Autodesk Inventor part; units mm, degrees
ref_plane "YZ Plane" through (0, 0, 0) normal (1, 0, 0) x (0, 1, 0)
ref_plane "XZ Plane" through (0, 0, 0) normal (0, 1, 0) x (-1, 0, 0)
ref_plane "XY Plane" through (0, 0, 0) normal (0, 0, 1) x (1, 0, 0)
sketch "Sketch1" plane through (0, 0, 0) normal (0, 0, 1) x (1, 0, 0)
  line L0 (0, 0) -> (-76.2, 0)
  line L1 (-76.2, 0) -> (-76.2, 3.175)
  line L2 (-76.2, 3.175) -> (-3.175, 3.175)
  line L3 (-3.175, 3.175) -> (-3.175, 53.975)
  line L4 (-3.175, 53.975) -> (0, 53.975)
  line L5 (0, 53.975) -> (0, 0)
  dimension "d0" = 76.2
  dimension "d1" = 50.8
  dimension "d2" = 3.175
extrude "Extrusion1" add sketch "Sketch1" along normal blind 60
sketch "Sketch2" plane through (-76.2, 3.175, 0) normal (0, 1, 0) x (1, 0, 0)
  line L0 (10.98, -50) -> (63.98, -50) construction
  line L1 (63.98, -50) -> (63.98, -10) construction
  line L2 (63.98, -10) -> (10.98, -10) construction
  line L3 (10.98, -10) -> (10.98, -50) construction
  line L4 (0, 0) -> (0, -60) construction
  line L5 (76.2, 0) -> (76.2, -60) construction
  circle A0 centre (10.98, -50) radius 2.5
  circle A1 centre (10.98, -10) radius 2.5
  circle A2 centre (63.98, -50) radius 2.5
  circle A3 centre (63.98, -10) radius 2.5
  point P0 (0, -30)
  point P1 (10.98, -30)
  dimension "d5" = 12.22
  dimension "d6" = 53
  dimension "d7" = 40
  dimension "d8" = 5
extrude "Extrusion2" cut sketch "Sketch2" against normal blind 60
properties part number "Z_Screw_Holder_Bracket"
Check sheet for the modelled part. Datum: model origin and axes. Units: mm. A direction names the side the tool comes from. Round coordinates to 2 decimals unless told otherwise and drop trailing zeros. Loops run counter-clockwise (first coordinate to the right, second up) from the corner with the lowest first, then second, coordinate; pieces in that order, holes last. Notation, with made-up numbers: (7.25, -20.5) - (21.25, -20.5) arc R21 cw to (21.25, 3.5) - close; hole circle Ø11 at (72, 2.5). An arc over 180 degrees is marked (long way). Answer as CSV lines item,"result". Start each with the question number.
Item 1: Set-up check for faces 1 (the flat face through (-2, 53.975, 30)), 2 (the flat face through (-40, 3.175, 30)): record each of +Z, -Z, +X, -X, +Y, -Y from which the full face is reachable in a straight line by a thin tool's end or side.
Item 2: Section check B-B (z = 10). Record the boundary of the cut face in (x, y) (3 decimals).
Item 3: Section check D-D (y = 22.5). Record the boundary of the cut face in (x, z) (3 decimals).
Item 4: Release check for a two-part mould opening along Z. For faces 3 (the flat face through (-27, 3, 60)), 4 (the cylindrical face through (-67.718, 1.61, 9.89)), 5 (the flat face through (-3.175, 28, 30)) record: +Z half, -Z half, draft (parallel to the pull), parting line (faces both ways), or undercut.
Item 5: Scan lines: line 1 (X direction, y = 2.4, z = 50); line 2 (Z direction, x = -65.22, y = 1.4); line 3 (X direction, y = 22.5, z = 23.5) (3 decimals). Record each from-to range of solid material in increasing order. Write a range as [from, to].
Item 6: Section check A-A (x = -65.22). Record the boundary of the cut face in (y, z) (3 decimals).
Item 7: Depth check by flat-ended pin: P1, Ø1.5, axis at y = 42, z = 34.5, coming from the -X side (3 decimals); P2, Ø6, axis at x = -12.22, z = 10, coming from the +Y side (3 decimals); P3, Ø8, axis at y = 15.5, z = 41, coming from the +X side; P4, Ø4.5, axis at x = -65.22, z = 10, coming from the -Y side. Enter the tip coordinate at first touch or a pass-through.
Item 8: Section check C-C (z = 19). Record the boundary of the cut face in (x, y) (3 decimals), and give its area (3 significant figures).
Report:
1,face 1,"+Z, -Z, +X, -X, +Y"
1,face 2,"+Z, -Z, -X, +Y"
2,outline,"(-76.2, 0) - (-67.72, 0) - (-67.72, 3.175) - (-76.2, 3.175) - close; (-62.72, 0) - (-14.72, 0) - (-14.72, 3.175) - (-62.72, 3.175) - close; (-9.72, 0) - (0, 0) - (0, 53.975) - (-3.175, 53.975) - (-3.175, 3.175) - (-9.72, 3.175) - close"
3,outline,"(-3.175, 0) - (0, 0) - (0, 60) - (-3.175, 60) - close"
4,face 3,"+Z half"
4,face 4,"undercut"
4,face 5,"draft"
5,line 1,"x = [-76.2, -67.72], [-62.72, -14.72], [-9.72, 0]"
5,line 2,"z = [0, 7.5], [12.5, 47.5], [52.5, 60]"
5,line 3,"x = [-3.175, 0]"
6,outline,"(0, 0) - (3.175, 0) - (3.175, 7.5) - (0, 7.5) - close; (0, 12.5) - (3.175, 12.5) - (3.175, 47.5) - (0, 47.5) - close; (0, 52.5) - (3.175, 52.5) - (3.175, 60) - (0, 60) - close"
7,P1,"stops at x = -3.175"
7,P2,"stops at y = 3.175"
7,P3,"stops at x = 0"
7,P4,"passes through"
8,outline,"(-76.2, 0) - (0, 0) - (0, 53.975) - (-3.175, 53.975) - (-3.175, 3.175) - (-76.2, 3.175) - close"
8,area,"403 mm2"
